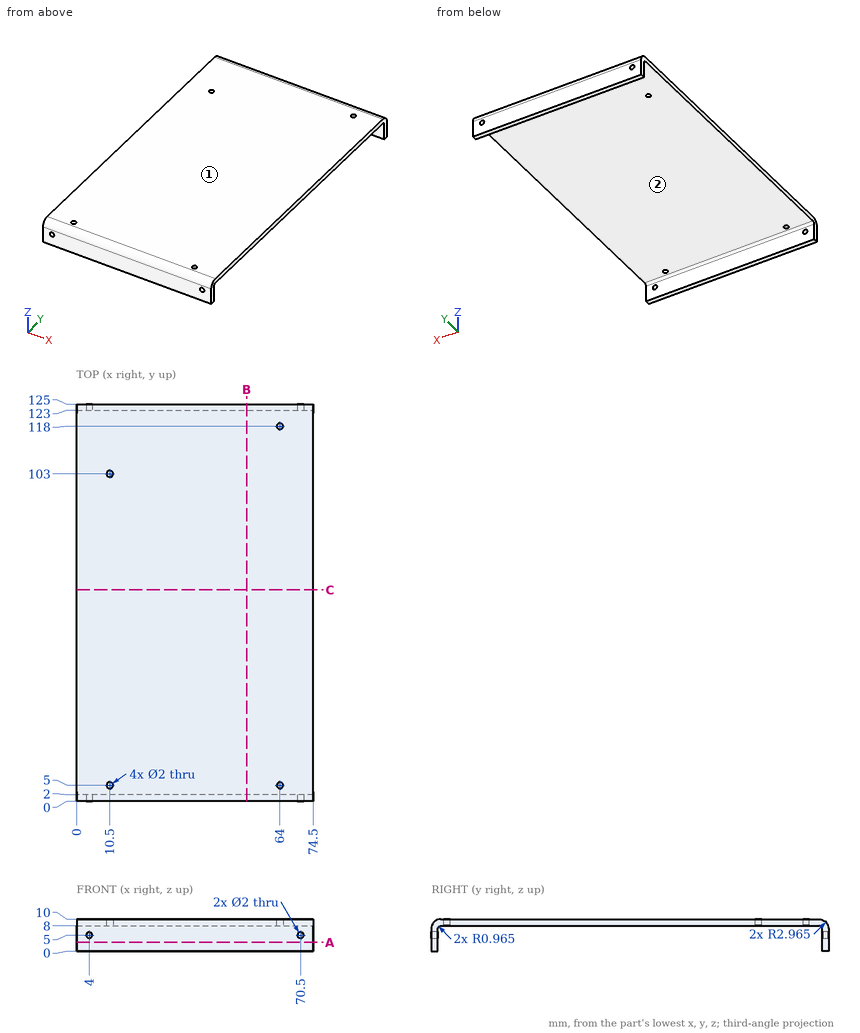
Input: dimensioned drawing with shaded views. Units: mm. Origin: part minimum x, y, z. Give positions to 0.01 mm unless a question says otherwise; leave off trailing zeros. Write each loop counter-clockwise with the first axis right and the second up, starting at its lowest first coordinate (ties: lowest second). Pieces come first, ordered by that corner, then holes. Notation, with made-up numbers: (71, 29) -> (100, 29) arc R15 cw to (100, 37) -> close; hole circle Ø5 at (-0.5, -39.5). An arc over 180 degrees is marked (long way). Return JSON: item names as keys, results as strings. Group by question number.
1. Mould query, pull axis Y, two halves, no side actions, for the marked faces 1 and 2. Classes: +Y half, -Y half, draft (parallel to the pull), parting line (faces both ways), or undercut.
2. Section B-B, the plane x = 53.5. Output: boundary loops of the cut face in (y, z) (1 decimal), then the cut area to 3 significant figures.
3. Section C-C, the plane y = 66.5. Output: boundary loops of the cut face in (x, z).
4. Pin query (flat end, axial travel): pin 1 Ø6 at (x, z) = (32.5, 9) entering from +Y; pin 2 Ø2.5 at (x, y) = (64, 5) entering from -Z. Return the tip coordinate at first contact, or that it passes through.
5. Material intervals for line 1 (X direction, y = 5, z = 8.45); line 2 (Y direction, x = 23, z = 6.5); line 3 (Y direction, x = 64, z = 8.65), sorted ascending. Write a range as from..to.
6. Section A-A, the plane z = 2.75. Output: boundary loops of the cut face in (x, y), then the cut area to 3 significant figures.
Determined:
{
 "1": {"face 1": "draft", "face 2": "undercut"},
 "2": {"outline": "(0, 0) -> (2, 0) -> (2, 7) arc R1 cw to (3, 8) -> (122, 8) arc R1 cw to (123, 7) -> (123, 0) -> (125, 0) -> (125, 7) arc R3 ccw to (122, 10) -> (3, 10) arc R3 ccw to (0, 7) -> close", "area": "279 mm2"},
 "3": {"outline": "(0, 8) -> (74.5, 8) -> (74.5, 10) -> (0, 10) -> close"},
 "4": {"pin 1": "stops at y = 125", "pin 2": "stops at z = 8"},
 "5": {"line 1": "x = 0..9.5, 11.5..63, 65..74.5", "line 2": "y = 0..2, 123..125", "line 3": "y = 0.48..4, 6..117, 119..124.52"},
 "6": {"outline": "(0, 0) -> (74.5, 0) -> (74.5, 2) -> (0, 2) -> close; (0, 123) -> (74.5, 123) -> (74.5, 125) -> (0, 125) -> close", "area": "298 mm2"}
}
